Verification items for the finished model (mm, model axes). A direction names the side the tool comes from. Round coordinates to 2 decimals unless told otherwise and drop trailing zeros. Write each loop counter-clockwise with the first axis right and the second up, starting at its lowest first coordinate (ties: lowest second). Pieces come first, ordered by that corner, then holes. Notation, with made-up numbers: (-11, -8.5) -> (45, -8.5) arc R22 ccw to (45, 4.5) -> close; hole circle Ø7 at (66.5, 4). An arc over 180 degrees is marked (long way). Answer as a JSON object with one key per item and string values. Group by question number.
(1) Sectioned sample at A-A on y = 2. Record the cut outline in (x, z).
(2) Draft check along Z on faces 1 (the face through (-5.51, 16.89, 2)), 2 (the face through (-11.07, 0.696, 15.985)), 3 (the face through (-11.1, 0.5, -15.8)). Enter one of: released by +Z, released by -Z, zero draft, split by the parting line, or undercut.
(3) Scan lines: L1, parallel to Y at x = -16.5, z = 16; L2, parallel to X at y = 11, z = -12; L3, parallel to X at y = 14, z = 16. Record each from-to range of solid material in increasing order. Write a range as from..to.
(4) Sectioned sample at C-C on x = -12. Record the cut outline in (y, z), and give its area (3 significant figures).
(5) Gauge pin test, flat ends, axial feed: pin 1 Ø3.5 at (x, z) = (-10.5, -16) entering from -Y; pin 2 Ø1.5 at (x, y) = (-10.5, 0) entering from +Z; pin 3 Ø6 at (x, z) = (-10, 8.5) entering from +Y (3 decimals). Record the tip position at first contact, or that the pin passes through.
(6) Set-up check for faces 4 (the face through (-5.507, 0.784, 17.983)), 5 (the face through (-16.5, -18, 8.9)), 6 (the face through (-16, -3, 16)), 7 (the face through (-11.1, -0.5, -15.8)): record each of +Z, -Z, +X, -X, +Y, -Y from which the full face is reachable in a straight line by a thin tool's end or side.
(7) Sectioned sample at B-B on z = 7. Record the cut outline in (x, y).
```python
from build123d import *

# Parameters (mm, degrees)
CYLINDER079_R     = 0.55
CYLINDER079_DEPTH = 12
CYLINDER078_R     = 0.55
CYLINDER078_DEPTH = 12
CYLINDER073_R     = 15
CYLINDER073_DEPTH = 12
CYLINDER072_R     = 1.1
CYLINDER072_DEPTH = 1
CYLINDER071_R     = 1.1
CYLINDER071_DEPTH = 1
BOX039_W          = 1
BOX039_H          = 36
BOX039_DEPTH      = 18
CYLINDER075_R     = 0.55
CYLINDER075_DEPTH = 12
CYLINDER074_R     = 0.55
CYLINDER074_DEPTH = 12
BOX038_W          = 12
BOX038_H          = 1
BOX038_DEPTH      = 5
CYLINDER069_R     = 16
CYLINDER069_DEPTH = 10
CYLINDER068_R     = 18
CYLINDER068_DEPTH = 10
CYLINDER067_R     = 15
CYLINDER067_DEPTH = 12
CYLINDER066_R     = 18
CYLINDER066_DEPTH = 12


with BuildPart() as zylinder076:
    # Cylinder079 → Cylinder079 (new body)
    with BuildSketch(Plane(origin=(-17, 16.11, 3.93), x_dir=(0, 0, -1), z_dir=(1, 0, 0))):
        Circle(CYLINDER079_R)
    extrude(amount=CYLINDER079_DEPTH)


with BuildPart() as fusion037:
    # Cylinder078 → Cylinder078 (new body)
    with BuildSketch(Plane(origin=(-17, 16.43, 2.3), x_dir=(0, 0, -1), z_dir=(1, 0, 0))):
        Circle(CYLINDER078_R)
    extrude(amount=CYLINDER078_DEPTH)

    # Fusion037: union Zylinder076
    add(zylinder076.part)


with BuildPart() as zylinder070:
    # Cylinder073 → Cylinder073 (new body)
    with BuildSketch(Plane(origin=(-17, 0, 0), x_dir=(0, 0, -1), z_dir=(1, 0, 0))):
        Circle(CYLINDER073_R)
    extrude(amount=CYLINDER073_DEPTH)


with BuildPart() as zylinder069:
    # Cylinder072 → Cylinder072 (new body)
    with BuildSketch(Plane(origin=(-17, 16, 16), x_dir=(0, 0, -1), z_dir=(1, 0, 0))):
        Circle(CYLINDER072_R)
    extrude(amount=CYLINDER072_DEPTH)


with BuildPart() as fusion034:
    # Cylinder071 → Cylinder071 (new body)
    with BuildSketch(Plane(origin=(-17, -16, 16), x_dir=(0, 0, -1), z_dir=(1, 0, 0))):
        Circle(CYLINDER071_R)
    extrude(amount=CYLINDER071_DEPTH)

    # Fusion034: union Zylinder069
    add(zylinder069.part)


with BuildPart() as cut059:
    # Box039 → Box039 (new body)
    with BuildSketch(Plane(origin=(-17, -18, 0), x_dir=(1, 0, 0), z_dir=(0, 0, 1))):
        with Locations((0.5, 18)):
            Rectangle(BOX039_W, BOX039_H)
    extrude(amount=BOX039_DEPTH)

    # Cut055: cut Fusion034
    add(fusion034.part, mode=Mode.SUBTRACT)

    # Cut056: cut Zylinder070
    add(zylinder070.part, mode=Mode.SUBTRACT)

    # Cut059: cut Fusion037
    add(fusion037.part, mode=Mode.SUBTRACT)


with BuildPart() as zylinder072:
    # Cylinder075 → Cylinder075 (new body)
    with BuildSketch(Plane(origin=(-17, 16.11, 3.93), x_dir=(0, 0, -1), z_dir=(1, 0, 0))):
        Circle(CYLINDER075_R)
    extrude(amount=CYLINDER075_DEPTH)


with BuildPart() as fusion035:
    # Cylinder074 → Cylinder074 (new body)
    with BuildSketch(Plane(origin=(-17, 16.43, 2.3), x_dir=(0, 0, -1), z_dir=(1, 0, 0))):
        Circle(CYLINDER074_R)
    extrude(amount=CYLINDER074_DEPTH)

    # Fusion035: union Zylinder072
    add(zylinder072.part)


with BuildPart() as obj1:
    # Box038 → Box038 (new body)
    with BuildSketch(Plane(origin=(-17, -0.5, -19), x_dir=(1, 0, 0), z_dir=(0, 0, 1))):
        with Locations((6, 0.5)):
            Rectangle(BOX038_W, BOX038_H)
    extrude(amount=BOX038_DEPTH)


with BuildPart() as zylinder066:
    # Cylinder069 → Cylinder069 (new body)
    with BuildSketch(Plane(origin=(0, 0, 0), x_dir=(0, 0, -1), z_dir=(1, 0, 0))):
        Circle(CYLINDER069_R)
    extrude(amount=CYLINDER069_DEPTH)


with BuildPart() as cut050:
    # Cylinder068 → Cylinder068 (new body)
    with BuildSketch(Plane(origin=(0, 0, 0), x_dir=(0, 0, -1), z_dir=(1, 0, 0))):
        Circle(CYLINDER068_R)
    extrude(amount=CYLINDER068_DEPTH)

    # Cut050: cut Zylinder066
    add(zylinder066.part, mode=Mode.SUBTRACT)


with BuildPart() as cut050_1:
    # Cut050 placement: moved
    add(cut050.part.moved(Location((-16, 0, 0))))


with BuildPart() as zylinder064:
    # Cylinder067 → Cylinder067 (new body)
    with BuildSketch(Plane(origin=(0, 0, 0), x_dir=(0, 0, -1), z_dir=(1, 0, 0))):
        Circle(CYLINDER067_R)
    extrude(amount=CYLINDER067_DEPTH)


with BuildPart() as fusion038:
    # Cylinder066 → Cylinder066 (new body)
    with BuildSketch(Plane(origin=(0, 0, 0), x_dir=(0, 0, -1), z_dir=(1, 0, 0))):
        Circle(CYLINDER066_R)
    extrude(amount=CYLINDER066_DEPTH)

    # Cut049: cut Zylinder064
    add(zylinder064.part, mode=Mode.SUBTRACT)


with BuildPart() as fusion038_1:
    # Cut049 placement: moved
    add(fusion038.part.moved(Location((-17, 0, 0))))

    # Cut051: cut Cut050
    add(cut050_1.part, mode=Mode.SUBTRACT)

    # Cut054: cut obj1
    add(obj1.part, mode=Mode.SUBTRACT)

    # Cut057: cut Fusion035
    add(fusion035.part, mode=Mode.SUBTRACT)

    # Fusion038: union Cut059
    add(cut059.part)


solid = fusion038_1.part
```
Computed values:
{
 "1": {"outline": "(-17, -17.89) -> (-16, -17.89) -> (-16, -15.87) -> (-6, -15.87) -> (-6, -17.89) -> (-5, -17.89) -> (-5, -14.87) -> (-17, -14.87) -> close; (-17, 14.87) -> (-5, 14.87) -> (-5, 17.89) -> (-6, 17.89) -> (-6, 15.87) -> (-16, 15.87) -> (-16, 18) -> (-17, 18) -> close"},
 "2": {"face 1": "undercut", "face 2": "split by the parting line", "face 3": "zero draft"},
 "3": {"L1": "-18..-17.1, -14.9..14.9, 17.1..18", "L2": "-17..-16, -6..-5", "L3": "-17..-16"},
 "4": {"outline": "(-0.5, -15.99) -> (-0.5, -14.99) arc R15 cw (long way) to (0.5, -14.99) -> (0.5, -15.99) arc R16 ccw (long way) to start", "area": "96.4 mm2"},
 "5": {"pin 1": "y = -7.28", "pin 2": "z = 16", "pin 3": "y = 15.025"},
 "6": {"face 4": "+X", "face 5": "+Z, -Z, +X, -X, -Y", "face 6": "none", "face 7": "-Z, +X, -X"},
 "7": {"outline": "(-17, -18) -> (-16, -18) -> (-16, -14.39) -> (-6, -14.39) -> (-6, -16.58) -> (-5, -16.58) -> (-5, -13.27) -> (-17, -13.27) -> close; (-17, 13.27) -> (-5, 13.27) -> (-5, 16.58) -> (-6, 16.58) -> (-6, 14.39) -> (-16, 14.39) -> (-16, 18) -> (-17, 18) -> close"}
}
